```python
from build123d import *

# Parameters (mm, degrees)
ESQUISSE1_W                           = 200
ESQUISSE1_H                           = 30
BOSS_EXTRU_1_DEPTH                    = 20
ESQUISSE2_W                           = 83
ESQUISSE2_H                           = 20
BOSS_EXTRU_2_DEPTH                    = 170
ESQUISSE3_W                           = 10
ESQUISSE3_H                           = 20
BOSS_EXTRU_3_DEPTH                    = 40
ESQUISSE4_W                           = 10
ESQUISSE4_H                           = 20
BOSS_EXTRU_4_DEPTH                    = 40
ESQUISSE5_W                           = 10
ESQUISSE5_H                           = 20
BOSS_EXTRU_5_DEPTH                    = 210
ESQUISSE6_W                           = 10
ESQUISSE6_H                           = 20
BOSS_EXTRU_6_DEPTH                    = 210
ENL_V_MAT_EXTRU_1_DEPTH               = 5
ESQUISSE8_W                           = 200
ESQUISSE8_H                           = 20
BOSS_EXTRU_7_DEPTH                    = 10
ESQUISSE9_W                           = 46.979991994
ESQUISSE9_H                           = 10
ENL_V_MAT_EXTRU_2_DEPTH               = 176.144775689
ESQUISSE10_W                          = 46.979991993
ESQUISSE10_H                          = 10
ENL_V_MAT_EXTRU_3_DEPTH               = 176.144775689
ESQUISSE11_W                          = 63
ESQUISSE11_H                          = 105.446
ENL_V_MAT_EXTRU_4_DEPTH               = 175.644474436
ESQUISSE12_W                          = 8
ESQUISSE12_H                          = 54.5
ENL_V_MAT_EXTRU_5_DEPTH               = 75.65
D_POUILLE1_ANGLE                      = 51.317812547
D_POUILLE2_ANGLE                      = 51.317812547
DIAM_TRE_DU_PER_AGE_4_2_4_2_1_D       = 4.2
DIAM_TRE_DU_PER_AGE_4_2_4_2_2_D       = 4.2
DIAM_TRE_DU_PER_AGE_4_2_4_2_2_DEPTH   = 20
DIAM_TRE_DU_PER_AGE_1_75_1_75_1_D     = 1.75
DIAM_TRE_DU_PER_AGE_1_75_1_75_1_DEPTH = 20
CHANFREIN1_SIZE                       = 12.489995997
CHANFREIN1_SIZE2                      = 10
CHANFREIN2_SIZE                       = 10
CHANFREIN2_SIZE2                      = 12.489995997
CHANFREIN3_SIZE                       = 4.803844614
CHANFREIN3_SIZE2                      = 6
CHANFREIN4_SIZE                       = 6
CHANFREIN4_SIZE2                      = 4.803844614


with BuildPart() as part:
    # Esquisse1 → Boss.-Extru.1 (new body)
    with BuildSketch(Plane.XY.offset(106.902665531)):
        with Locations((-11.355880004, -118.699515481)):
            Rectangle(ESQUISSE1_W, ESQUISSE1_H)
    extrude(amount=-BOSS_EXTRU_1_DEPTH)

    # Esquisse2 → Boss.-Extru.2 (add)
    with BuildSketch(Plane(origin=(0, -103.699515481, 0), x_dir=(-1, 0, 0), z_dir=(0, 1, 0))):
        with Locations((11.355880004, 96.902665531)):
            Rectangle(ESQUISSE2_W, ESQUISSE2_H)
    extrude(amount=BOSS_EXTRU_2_DEPTH)

    # Esquisse3 → Boss.-Extru.3 (add)
    with BuildSketch(Plane(origin=(0, 66.300484519, 0), x_dir=(-1, 0, 0), z_dir=(0, 1, 0))):
        with Locations((-25.144119996, 96.902665531)):
            Rectangle(ESQUISSE3_W, ESQUISSE3_H)
    extrude(amount=BOSS_EXTRU_3_DEPTH)

    # Esquisse4 → Boss.-Extru.4 (add)
    with BuildSketch(Plane(origin=(0, 66.300484519, 0), x_dir=(-1, 0, 0), z_dir=(0, 1, 0))):
        with Locations((47.855880004, 96.902665531)):
            Rectangle(ESQUISSE4_W, ESQUISSE4_H)
    extrude(amount=BOSS_EXTRU_4_DEPTH)

    # Esquisse5 → Boss.-Extru.5 (add)
    with BuildSketch(Plane(origin=(0, -103.699515481, 0), x_dir=(-1, 0, 0), z_dir=(0, 1, 0))):
        with Locations((-83.644119996, 96.902665531)):
            Rectangle(ESQUISSE5_W, ESQUISSE5_H)
    extrude(amount=BOSS_EXTRU_5_DEPTH)

    # Esquisse6 → Boss.-Extru.6 (add)
    with BuildSketch(Plane(origin=(0, -103.699515481, 0), x_dir=(-1, 0, 0), z_dir=(0, 1, 0))):
        with Locations((106.355880004, 96.902665531)):
            Rectangle(ESQUISSE6_W, ESQUISSE6_H)
    extrude(amount=BOSS_EXTRU_6_DEPTH)

    # Esquisse7 → Enlèv. mat.-Extru.1 (cut)
    with BuildSketch(Plane.XY.offset(106.902665531)):
        Polygon((-42.855880004, 106.300484519), (-52.855880004, 106.300484519), (-52.855880004, -103.699515481), (-101.355880004, -103.699515481), (-101.355880004, -113.699515481), (-60.865884007, -113.699515481), (-60.865884007, -123.699515481), (38.154124, -123.699515481), (38.154124, -113.699515481), (78.644119996, -113.699515481), (78.644119996, -103.699515481), (30.144119996, -103.699515481), (30.144119996, 106.300484519), (20.144119996, 106.300484519), (20.144119996, 66.300484519), (-42.855880004, 66.300484519), align=None)
    extrude(amount=-ENL_V_MAT_EXTRU_1_DEPTH, mode=Mode.SUBTRACT)

    # Esquisse8 → Boss.-Extru.7 (add)
    with BuildSketch(Plane(origin=(0, 106.300484519, 0), x_dir=(-1, 0, 0), z_dir=(0, 1, 0))):
        with Locations((11.355880004, 96.902665531)):
            Rectangle(ESQUISSE8_W, ESQUISSE8_H)
    extrude(amount=BOSS_EXTRU_7_DEPTH)

    # Esquisse9 → Enlèv. mat.-Extru.2 (cut, through all)
    with BuildSketch(Plane(origin=(0, 0, 86.902665531), x_dir=(-1, 0, 0), z_dir=(0, 0, -1))):
        with Locations((87.865884007, -128.699515481)):
            Rectangle(ESQUISSE9_W, ESQUISSE9_H)
    extrude(amount=-ENL_V_MAT_EXTRU_2_DEPTH, mode=Mode.SUBTRACT)

    # Esquisse10 → Enlèv. mat.-Extru.3 (cut, through all)
    with BuildSketch(Plane(origin=(0, 0, 86.902665531), x_dir=(-1, 0, 0), z_dir=(0, 0, -1))):
        with Locations((-65.154124, -128.699515481)):
            Rectangle(ESQUISSE10_W, ESQUISSE10_H)
    extrude(amount=-ENL_V_MAT_EXTRU_3_DEPTH, mode=Mode.SUBTRACT)

    # Esquisse11 → Enlèv. mat.-Extru.4 (cut, through all)
    with BuildSketch(Plane.XY.offset(101.902665531)):
        with Locations((-11.355880004, -50.976515481)):
            Rectangle(ESQUISSE11_W, ESQUISSE11_H)
    extrude(amount=-ENL_V_MAT_EXTRU_4_DEPTH, mode=Mode.SUBTRACT)

    # Esquisse12 → Enlèv. mat.-Extru.5 (cut)
    with BuildSketch(Plane.ZY.offset(52.855880004)):
        with Locations((97.902665531, 34.023484519)):
            Rectangle(ESQUISSE12_W, ESQUISSE12_H)
    extrude(amount=-ENL_V_MAT_EXTRU_5_DEPTH, mode=Mode.SUBTRACT)

    # Dépouille1
    d_pouille1_faces = [part.faces().sort_by_distance(p)[0] for p in [
        (38.154124, -118.699515481, 104.402665531),
        (-60.865884007, -118.699515481, 104.402665531),
    ]]
    draft(d_pouille1_faces, Plane(origin=(-60.865884007, -123.699515481, 101.902665531), x_dir=(0, 0, 1), z_dir=(0, 1, 0)), D_POUILLE1_ANGLE)

    # Dépouille2
    d_pouille2_faces = [part.faces().sort_by_distance(p)[0] for p in [
        (41.664128003, -128.699515481, 96.902665531),
        (-64.37588801, -128.699515481, 96.902665531),
    ]]
    draft(d_pouille2_faces, Plane(origin=(-111.355880004, -133.699515481, 86.902665531), x_dir=(-1, 0, 0), z_dir=(0, -1, 0)), D_POUILLE2_ANGLE)

    # Diamètre du perçage Ø4.2 (4.2)1 (through all)
    with Locations(Plane(origin=(0, 0, 86.902665531), x_dir=(-1, 0, 0), z_dir=(0, 0, -1))):
        with Locations((-73.644119996, -118.699515481), (96.355880004, -118.699515481), (106.330817189, 111.800484519), (-83.619057182, 111.800484519)):
            Hole(DIAM_TRE_DU_PER_AGE_4_2_4_2_1_D / 2)

    # Diamètre du perçage Ø4.2 (4.2)2
    with Locations(Plane(origin=(0, 0, 86.902665531), x_dir=(-1, 0, 0), z_dir=(0, 0, -1))):
        with Locations((47.855880004, -15.976515481), (-25.144119996, -15.976515481), (-25.144119996, 84.023484519), (47.855880004, 84.023484519)):
            Hole(DIAM_TRE_DU_PER_AGE_4_2_4_2_2_D / 2, depth=DIAM_TRE_DU_PER_AGE_4_2_4_2_2_DEPTH)

    # Diamètre du perçage Ø1.75 (1.75)1
    with Locations(Plane(origin=(0, 0, 86.902665531), x_dir=(-1, 0, 0), z_dir=(0, 0, -1))):
        with Locations((9.125880004, 9.253484519), (-20.564119996, 34.023484519), (9.125880004, 58.793484519)):
            Hole(DIAM_TRE_DU_PER_AGE_1_75_1_75_1_D / 2, depth=DIAM_TRE_DU_PER_AGE_1_75_1_75_1_DEPTH)

    # Chanfrein1
    chanfrein1_edges = [part.edges().sort_by_distance(p)[0] for p in [
        (88.644119996, -123.699515481, 96.902665531),
    ]]
    chanfrein1_side = [part.faces().sort_by_distance(p)[0] for p in [
        (71.399121998, -123.699515481, 96.902665531),
    ]]
    chamfer(chanfrein1_edges, length=CHANFREIN1_SIZE, length2=CHANFREIN1_SIZE2, reference=chanfrein1_side[0])

    # Chanfrein2
    chanfrein2_edges = [part.edges().sort_by_distance(p)[0] for p in [
        (-111.355880004, -123.699515481, 96.902665531),
    ]]
    chanfrein2_side = [part.faces().sort_by_distance(p)[0] for p in [
        (-111.355880004, -3.699515481, 96.902665531),
    ]]
    chamfer(chanfrein2_edges, length=CHANFREIN2_SIZE, length2=CHANFREIN2_SIZE2, reference=chanfrein2_side[0])

    # Chanfrein3
    chanfrein3_edges = [part.edges().sort_by_distance(p)[0] for p in [
        (-101.355880004, -113.699515481, 104.402665531),
    ]]
    chanfrein3_side = [part.faces().sort_by_distance(p)[0] for p in [
        (-101.355880004, 0.006366872, 96.990900825),
    ]]
    chamfer(chanfrein3_edges, length=CHANFREIN3_SIZE, length2=CHANFREIN3_SIZE2, reference=chanfrein3_side[0])

    # Chanfrein4
    chanfrein4_edges = [part.edges().sort_by_distance(p)[0] for p in [
        (78.644119996, -113.699515481, 104.402665531),
    ]]
    chanfrein4_side = [part.faces().sort_by_distance(p)[0] for p in [
        (64.644119996, -113.699515481, 104.402665531),
    ]]
    chamfer(chanfrein4_edges, length=CHANFREIN4_SIZE, length2=CHANFREIN4_SIZE2, reference=chanfrein4_side[0])


solid = part.part
```
The listing builds one solid part. Answer for the finished solid, in the listing's coordinates (mm). A direction names the side the tool comes from. Round coordinates to 2 decimals unless told otherwise and drop trailing zeros. Loops run counter-clockwise (first coordinate to the right, second up) from the corner with the lowest first, then second, coordinate; pieces in that order, holes last. Notation, with made-up numbers: (-36, 18) - (9, 18) arc R26 ccw to (9, 54) - close; hole circle Ø6 at (56, 27). An arc over 180 degrees is marked (long way). Return JSON: item names as keys, results as strings. Group by question number.
1. The part is cut by section D-D on x = -88. Determine the outline of the cut face in (y, z), then the cut area to 3 significant figures.
2. Each of these flat-tipped pins is pushed along its axis until it touches: P1, Ø10, axis at x = 63, z = 101, coming from the -Y side; P2, Ø5.5, axis at x = 73.64, y = -118.7, coming from the +Z side. Where does it stop, or does it pass through?
3. The part is cut by section C-C on y = 42.5. Determine the outline of the cut face in (x, z), then the cut area to 3 significant figures.
4. Consider probe 1 along Y at (x, z) = (18, 101.25); probe 2 along X at (y, z) = (-75, 98.75); probe 3 along X at (y, z) = (39.5, 96.75). Determine where each line is inside the solid, lowest interval first.
5. The part is cut by section B-B on y = -73.5. Determine the outline of the cut face in (x, z).
6. The part is cut by section A-A on x = -17.5. Determine the outline of the cut face in (y, z), then the cut area to 3 significant figures.
7. Which of the six approach directions +Z, -Z, +X, -X, +Y, -Y give full straight-line access (tool end or side, diameter ignored) to faces 1 (the flat face through (-88, -123.7, 97)), 2 (the flat face through (30.144, 0, 94)), 3 (the flat face through (85, -19, 106.903)), 4 (the flat face through (44.31, -118.77, 104.44))?
8. The mould has two halves that part along Y. Classify faces 5 (the flat face through (65, -123.7, 97)), 6 (the flat face through (-111.356, 0, 97)), 7 (the flat face through (22, -42, 101.903)): pulls with the +Y half, pulls with the -Y half, needs draft (parallel to the pull), parting line crosses it, or undercut.
Resolved:
{
 "1": {"outline": "(-123.7, 86.9) - (-103.7, 86.9) - (-103.7, 101.9) - (-113.7, 101.9) - (-113.7, 106.9) - (-123.7, 106.9) - close; (106.3, 86.9) - (116.3, 86.9) - (116.3, 106.9) - (106.3, 106.9) - close", "area": "550 mm²"},
 "2": {"P1": "stops at y = -123.7", "P2": "stops at z = 106.9"},
 "3": {"outline": "(-111.36, 86.9) - (-101.36, 86.9) - (-101.36, 106.9) - (-111.36, 106.9) - close; (-52.86, 86.9) - (30.14, 86.9) - (30.14, 101.9) - (22.79, 101.9) - (22.79, 93.9) - (-52.86, 93.9) - close; (78.64, 86.9) - (88.64, 86.9) - (88.64, 106.9) - (78.64, 106.9) - close", "area": "1,040 mm²"},
 "4": {"probe 1": "y = -133.7 to -103.7, 1.75 to 6.77, 61.27 to 66.3, 106.3 to 116.3", "probe 2": "x = -111.36 to -101.36, -52.86 to -42.86, 20.14 to 30.14, 78.64 to 88.64", "probe 3": "x = -111.36 to -101.36, 22.79 to 30.14, 78.64 to 88.64"},
 "5": {"outline": "(-111.36, 86.9) - (-101.36, 86.9) - (-101.36, 106.9) - (-111.36, 106.9) - close; (-52.86, 86.9) - (-42.86, 86.9) - (-42.86, 101.9) - (-52.86, 101.9) - close; (20.14, 86.9) - (30.14, 86.9) - (30.14, 101.9) - (20.14, 101.9) - close; (78.64, 86.9) - (88.64, 86.9) - (88.64, 106.9) - (78.64, 106.9) - close"},
 "6": {"outline": "(-133.7, 86.9) - (-103.7, 86.9) - (-103.7, 101.9) - (-123.7, 101.9) - (-123.7, 106.9) - (-133.7, 106.9) - close; (1.75, 86.9) - (66.3, 86.9) - (66.3, 101.9) - (61.27, 101.9) - (61.27, 93.9) - (6.77, 93.9) - (6.77, 101.9) - (1.75, 101.9) - close; (106.3, 86.9) - (116.3, 86.9) - (116.3, 106.9) - (106.3, 106.9) - close", "area": "1,230 mm²"},
 "7": {"face 1": "+Z, -Z, -X, -Y", "face 2": "+Z, -Z", "face 3": "+Z, +X, -X, +Y, -Y", "face 4": "+Z"},
 "8": {"face 5": "pulls with the -Y half", "face 6": "needs draft", "face 7": "undercut"}
}
